Read the model definition and answer for the solid it produces. Units are mm, in the model's axes. A direction names the side the tool comes from. Round coordinates to 2 decimals unless told otherwise and drop trailing zeros. Order: outer loops, then holes, each group sorted by start corner. A loop starts at its lowest first (then second) coordinate and runs counter-clockwise, first axis right, second up. Notation, with made-up numbers: (33.25, 4.25) -> (62.25, 4.25) arc R31 ccw to (62.25, 33.25) -> close; hole circle Ø10 at (57, 18.25). An arc over 180 degrees is marked (long way). Use a Markdown table: item, result. Add a question column.
1. The mould has two halves that part along Y. Classify faces 3 (the face through (375.666, 1320.775, -2.234)), 4 (the face through (375.666, -101.575, 2.234)), 5 (the face through (375.67, 1295.38, 1.68)), 6 (the face through (762, 606, 83)): +Y half, -Y half, draft (parallel to the pull), parting line (faces both ways), or undercut.
2. Section B-B, the plane z = 0 is taken. Give the vertices of the cut face in (x, y).
3. Section C-C, the plane x = 338.5 is taken. Give the vertices of the cut face in (y, z), then the cut area to 3 significant figures.
4. Consider L1, parallel to Z at x = 360.5, y = 964; L2, parallel to Y at x = 61.5, z = 6.5; L3, parallel to Y at x = 628, z = -55. Determine where each line is inside the solid, lowest interval first. Write a range as [from, to].
5. Section A-A, the plane y = 247.5 is taken. Give the vertices of the cut face in (x, z), then the cut area to 3 significant figures.
6. For faces 1 (the face through (0, 606, 83)), 2 (the face through (376, 601, 76.2)), determine the directions among +Z, -Z, +X, -X, +Y, -Y from which every point of the face is accessible in a straight line to the end or side of a thin tool.
7. Given pin 1 (2 mm diameter, centred on x = 495.5, z = 71, fed in from +Y); pin 2 (5 mm diameter, centred on x = 181, z = 31, fed in from -Y); pin 3 (6 mm diameter, centred on x = 126, z = 22.5, fed in from +Y), each flat-ended and moving along its own axis, determine where each tip first touches the part or whether it passes through.
```python
from build123d import *

# Parameters (mm, degrees)
F1_DEPTH = 762


with BuildPart() as f1:
    # F0 (on Right) → F1 (new body)
    with BuildSketch(Plane.YZ):
        with BuildLine():
            ThreePointArc((0, 76.2), (-76.2, 0), (0, -76.2))
            Line((0, -76.2), (1219.2, -76.2))
            ThreePointArc((1219.2, -76.2), (1295.4, 0), (1219.2, 76.2))
            Line((1219.2, 76.2), (0, 76.2))
        make_face()
        with BuildLine():
            ThreePointArc((0, 101.6), (-101.6, 0), (0, -101.6))
            Line((0, -101.6), (1219.2, -101.6))
            ThreePointArc((1219.2, -101.6), (1320.8, 0), (1219.2, 101.6))
            Line((1219.2, 101.6), (0, 101.6))
        make_face()
        with BuildLine():
            Line((1219.2, -76.2), (0, -76.2))
            ThreePointArc((0, -76.2), (-76.2, 0), (0, 76.2))
            Line((0, 76.2), (1219.2, 76.2))
            ThreePointArc((1219.2, 76.2), (1295.4, 0), (1219.2, -76.2))
        make_face(mode=Mode.SUBTRACT)
    extrude(amount=F1_DEPTH)


solid = f1.part
```
Verdict:
| question | item | result |
|---|---|---|
| 1 | face 3 | +Y half |
| 1 | face 4 | -Y half |
| 1 | face 5 | undercut |
| 1 | face 6 | draft |
| 2 | outline | (0, -101.6) -> (762, -101.6) -> (762, -76.2) -> (0, -76.2) -> close; (0, 1295.4) -> (762, 1295.4) -> (762, 1320.8) -> (0, 1320.8) -> close |
| 3 | outline | (0, -101.6) -> (1219.2, -101.6) arc R101.6 ccw to (1219.2, 101.6) -> (0, 101.6) arc R101.6 ccw to start; hole (0, -76.2) -> (1219.2, -76.2) arc R76.2 ccw to (1219.2, 76.2) -> (0, 76.2) arc R76.2 ccw to start |
| 3 | area | 76,100 mm2 |
| 4 | L1 | z = [-101.6, -76.2], [76.2, 101.6] |
| 4 | L2 | y = [-101.39, -75.92], [1295.12, 1320.59] |
| 4 | L3 | y = [-85.43, -52.74], [1271.94, 1304.63] |
| 5 | outline | (0, -101.6) -> (762, -101.6) -> (762, -76.2) -> (0, -76.2) -> close; (0, 76.2) -> (762, 76.2) -> (762, 101.6) -> (0, 101.6) -> close |
| 5 | area | 38,700 mm2 |
| 6 | face 1 | +Z, -Z, -X, +Y, -Y |
| 6 | face 2 | +X, -X |
| 7 | pin 1 | stops at y = 1292.84 |
| 7 | pin 2 | stops at y = -97.52 |
| 7 | pin 3 | stops at y = 1318.91 |
